Input: part model. Units: mm. Frame: model coordinates. Face numbers are marked on the shaded views. A direction names the side the tool comes from. Round coordinates to 2 decimals unless told otherwise and drop trailing zeros. Loops run counter-clockwise (first coordinate to the right, second up) from the corner with the lowest first, then second, coordinate; pieces in that order, holes last. Notation, with made-up numbers: M 59,10.25 L 66,10.25 A29 ccw 66,45.25 Z; hole C 12,38.25 d1. An arc over 180 degrees is marked long. Use one line per item in the form item = value. Start each with the question number.
Q1. Section query A-A, the plane y = 0. State how many separate pieces and enclosed holes the cut face has, and give its area (3 significant figures).
Q2. Access query for the marked faces 1, 2 and 3. Directions: +Z, -Z, +X, -X, +Y, -Y. A direction counts if a zero-diameter tool reaches every point of the face in a straight line with its end or side. Return the directions, or none.
Q3. Section query D-D, the plane x = -6.25. Output: boundary loops of the cut face in (y, z), and give its area (3 significant figures).
Q4. Ray query, line 1 along Z through (x, y) = (0, -9.45); line 2 along X through (y, z) = (-8, 20.5); line 3 along Y through (x, z) = (5, 4). Return the intervals inside material, ascending.
Q5. Mould query, pull axis Z, two halves, no side actions, for the marked faces 4, 5 and 6. Classes: pulls with the +Z half, pulls with the -Z half, needs draft (parallel to the pull), parting line crosses it, or undercut.
Q6. Section query B-B, the plane y = 10. Output: boundary loops of the cut face in (x, z), and give its area (3 significant figures).
Q7. First-contact query: P1, Ø3.5, axis at x = -6.25, y = -10.83, coming from the +Z side; P2, Ø5, axis at x = 0, z = 19.05, coming from the +Y side; P3, Ø4, axis at x = 2.5, z = 9.5, coming from the -Y side. Flat tips, straight axial feed; report the tip coordinate or a pass-through.
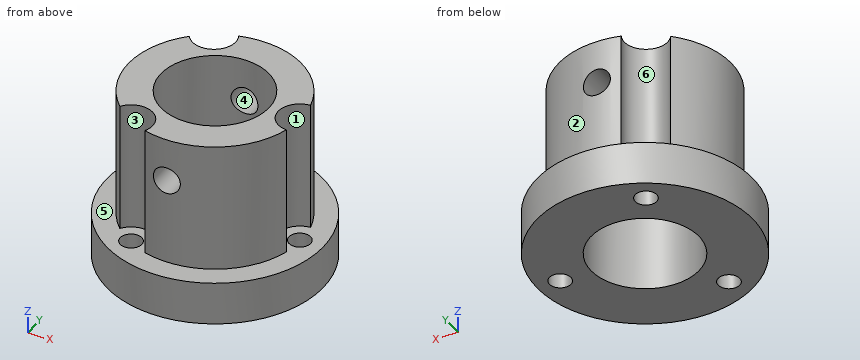
```python
from build123d import *

# Parameters (mm, degrees)
SKETCH1_R                           = 15.875
SKETCH1_R_2                         = 7.9375
BOSS_EXTRUDE1_DEPTH                 = 6.35
SKETCH2_R                           = 14.29
SKETCH2_R_2                         = 7.9375
BOSS_EXTRUDE2_DEPTH                 = 19.05
SKETCH3_R                           = 1.5875
CUT_EXTRUDE1_DEPTH                  = 14.8
CUT_EXTRUDE3_DEPTH                  = 34.89972345
CUT_EXTRUDE3_DEPTH_BACK             = 34.89972345
SKETCH4_R                           = 1.9844
SKETCH5_R                           = 3.175
CUT_EXTRUDE4_DEPTH                  = 19.05
CUT_START                           = -19.05
CUT_CHANGE_FROM_065_WT_TO_125_DEPTH = 19.05


# Read off the part's stored shape, not the designer's step: Cut- Change from .065 WT to .125
with BuildPart() as part:
    # Sketch1 → Boss-Extrude1 (new body)
    with BuildSketch(Plane.XY):
        Circle(SKETCH1_R)
        Circle(SKETCH1_R_2, mode=Mode.SUBTRACT)
    extrude(amount=BOSS_EXTRUDE1_DEPTH)

    # Sketch2 → Boss-Extrude2 (add)
    with BuildSketch(Plane.XY.offset(6.35)):
        Circle(SKETCH2_R)
        Circle(SKETCH2_R_2, mode=Mode.SUBTRACT)
    extrude(amount=BOSS_EXTRUDE2_DEPTH)

    # Sketch3 → Cut-Extrude1 (cut)
    with BuildSketch(Plane(origin=(0, 0, 0), x_dir=(-1, 0, 0), z_dir=(0, 0, -1))):
        with Locations((6.25, 10.825317547)):
            Circle(SKETCH3_R)
        with Locations((6.25, -10.825317547)):
            Circle(SKETCH3_R)
        with Locations((-12.5, 0)):
            Circle(SKETCH3_R)
    extrude(amount=-CUT_EXTRUDE1_DEPTH, mode=Mode.SUBTRACT)

    # Sketch4 → Cut-Extrude3 (cut, two sides: drawn at the far end of the back side and taken through both)
    with BuildSketch(Plane(origin=(0, 0, 0), x_dir=(1, 0, 0), z_dir=(0, 1, 0)).offset(-CUT_EXTRUDE3_DEPTH_BACK)):
        with Locations(Location((0, -19.05, 0), (0, 0, 270))):
            Circle(SKETCH4_R)
    extrude(amount=CUT_EXTRUDE3_DEPTH + CUT_EXTRUDE3_DEPTH_BACK, mode=Mode.SUBTRACT)

    # Sketch5 → Cut-Extrude4 (cut)
    with BuildSketch(Plane.XY.offset(25.4)):
        with Locations((-6.25, 10.825317547)):
            Circle(SKETCH5_R)
        with Locations((12.5, 0)):
            Circle(SKETCH5_R)
        with Locations((-6.25, -10.825317547)):
            Circle(SKETCH5_R)
    extrude(amount=-CUT_EXTRUDE4_DEPTH, mode=Mode.SUBTRACT)

    # Cut- Change from .065 WT to .125 outline → Cut- Change from .065 WT to .125 (cut)
    with BuildSketch(Plane.XY.offset(25.4).offset(CUT_START)):
        with BuildLine():
            ThreePointArc((-8.893268269, -9.066409404), (-12.7, 0), (-8.893268269, 9.066409404))
            ThreePointArc((-8.893268269, 9.066409404), (-9.276867733, 9.866830861), (-9.423910813, 10.742160164))
            ThreePointArc((-9.423910813, 10.742160164), (-14.29, 0), (-9.423910813, -10.742160164))
            ThreePointArc((-9.423910813, -10.742160164), (-9.276867733, -9.866830861), (-8.893268269, -9.066409404))
        make_face()
        with BuildLine():
            ThreePointArc((-4.591028187, 13.532426249), (-3.906492314, 12.967418555), (-3.405106731, 12.235000946))
            ThreePointArc((-3.405106731, 12.235000946), (6.35, 10.998522628), (12.298375, 3.168591542))
            ThreePointArc((12.298375, 3.168591542), (13.183360047, 3.100587694), (14.014939, 2.790266085))
            ThreePointArc((14.014939, 2.790266085), (7.145, 12.37550302), (-4.591028187, 13.532426249))
        make_face()
        with BuildLine():
            ThreePointArc((12.298375, -3.168591542), (6.35, -10.998522628), (-3.405106731, -12.235000946))
            ThreePointArc((-3.405106731, -12.235000946), (-3.906492314, -12.967418555), (-4.591028187, -13.532426249))
            ThreePointArc((-4.591028187, -13.532426249), (7.145, -12.37550302), (14.014939, -2.790266085))
            ThreePointArc((14.014939, -2.790266085), (13.183360047, -3.100587694), (12.298375, -3.168591542))
        make_face()
    extrude(amount=CUT_CHANGE_FROM_065_WT_TO_125_DEPTH, mode=Mode.SUBTRACT)


solid = part.part
```
Results found:
q1.separate_pieces = 3
q1.enclosed_holes = 0
q1.area = 198 mm²
q2.face_1 = +Z, +X
q2.face_2 = +Z, +Y
q2.face_3 = +Z
q3.outline = M -14.59,0 L -12.41,0 L -12.41,6.35 L -14.59,6.35 Z; M -9.24,0 L -4.89,0 L -4.89,25.4 L -7.65,25.4 L -7.65,6.35 L -9.24,6.35 Z; M 4.89,0 L 9.24,0 L 9.24,6.35 L 7.65,6.35 L 7.65,25.4 L 4.89,25.4 Z; M 12.41,0 L 14.59,0 L 14.59,6.35 L 12.41,6.35 Z
q3.area = 188 mm²
q4.line_1 = 0 to 17.07, 21.03 to 25.4
q4.line_2 = -9.86 to -7.7, -4.8 to -1.35, 1.35 to 9.86
q4.line_3 = -15.07 to -6.16, 6.16 to 15.07
q5.face_4 = undercut
q5.face_5 = pulls with the +Z half
q5.face_6 = needs draft
q6.outline = M -12.33,0 L -7.61,0 L -7.61,6.35 L -12.33,6.35 Z; M -4.89,0 L 12.33,0 L 12.33,6.35 L 7.83,6.35 L 7.83,25.4 L -3.18,25.4 L -3.18,6.35 L -4.89,6.35 Z; hole C 0,19.05 d3.97
q6.area = 337 mm²
q7.P1 = 6.35
q7.P2 = 12.7
q7.P3 = -12.69
